```python
from build123d import *
from OCP.BRepFilletAPI import BRepFilletAPI_MakeChamfer

# Parameters (mm, degrees)
SKETCH1_R                = 2.75
BOSS_EXTRUDE1_DEPTH      = 25
CUT_EXTRUDE1_DEPTH       = 37.486298798
CUT_EXTRUDE1_DEPTH_BACK  = 37.486298798
CUT_EXTRUDE2_START       = -5
SKETCH3_R                = 6
CUT_EXTRUDE2_DEPTH       = 28.113081447
CUT_EXTRUDE3_START       = -23.75
CUT_EXTRUDE3_DEPTH       = 23.75
CUT_EXTRUDE3_START_2     = -14.426375
CUT_EXTRUDE3_2_OUTLINE_R = 2
CUT_EXTRUDE3_2_DEPTH     = 14.426375
CHAMFER1_SIZE            = 2
CHAMFER1_SIZE2           = 7.211102551
CHAMFER2_SIZE            = 0.4
SKETCH5_W                = 6
SKETCH5_H                = 4
SKETCH5_W_2              = 4
SKETCH5_H_2              = 6
BOSS_EXTRUDE2_DEPTH      = 2
CHAMFER3_SIZE            = 2


with BuildPart() as part:
    # Sketch1 → Boss-Extrude1 (new body)
    with BuildSketch(Plane.XY):
        Polygon((-10, 10), (10, 10), (10, -10), (10, -17.5), (-10, -17.5), (-10, -10), align=None)
        Circle(SKETCH1_R, mode=Mode.SUBTRACT)
    extrude(amount=BOSS_EXTRUDE1_DEPTH)

    # Sketch2 → Cut-Extrude1 (cut, two sides: drawn at the far end of the back side and taken through both)
    with BuildSketch(Plane(origin=(10, 0, 0), x_dir=(0, 0, -1), z_dir=(1, 0, 0)).offset(-CUT_EXTRUDE1_DEPTH_BACK)):
        Polygon((-5, -17.5), (0, -10), (0, -17.5), align=None)
        Polygon((-12.5, 10), (-25, -8.75), (-25, 10), align=None)
    extrude(amount=CUT_EXTRUDE1_DEPTH + CUT_EXTRUDE1_DEPTH_BACK, mode=Mode.SUBTRACT)

    # Sketch3 → Cut-Extrude2 (cut, through all)
    with BuildSketch(Plane(origin=(0, 0, 0), x_dir=(-1, 0, 0), z_dir=(0, 0, -1)).offset(CUT_EXTRUDE2_START)):
        Circle(SKETCH3_R)
    extrude(amount=-CUT_EXTRUDE2_DEPTH, mode=Mode.SUBTRACT)

    # Cut-Extrude3: read off the stored shape, not the designer's step
    # Cut-Extrude3 outline → Cut-Extrude3 (cut)
    with BuildSketch(Plane.XZ.offset(17.5).offset(CUT_EXTRUDE3_START)):
        with BuildLine():
            ThreePointArc((-10, 15), (-7.071067812, 22.071067812), (0, 25))
            Line((0, 25), (-10, 25))
            Line((-10, 25), (-10, 15))
        make_face()
        with BuildLine():
            ThreePointArc((0, 25), (7.071067812, 22.071067812), (10, 15))
            Line((10, 15), (10, 25))
            Line((10, 25), (0, 25))
        make_face()
    extrude(amount=CUT_EXTRUDE3_DEPTH, mode=Mode.SUBTRACT)

    # Cut-Extrude3 2 outline → Cut-Extrude3 2 (cut)
    with BuildSketch(Plane.XZ.offset(17.5).offset(CUT_EXTRUDE3_START_2)):
        with Locations((0, 15)):
            Circle(CUT_EXTRUDE3_2_OUTLINE_R)
    extrude(amount=CUT_EXTRUDE3_2_DEPTH, mode=Mode.SUBTRACT)

    # Chamfer1: one chamfer whose edges measure the first distance from different faces: ONE call of the kernel's chamfer builder (chamfer() names one face for all edges)
    chamfer1_edges_1 = [part.edges().sort_by_distance(p)[0] for p in [
        (-10, 10, 6.25),
        (10, 10, 6.25),
    ]]
    chamfer1_edges_2 = [part.edges().sort_by_distance(p)[0] for p in [
        (0, 10, 12.5),
    ]]
    chamfer1_side_2 = [part.faces().sort_by_distance(p)[0] for p in [
        (-9.69870073, 8.125, 13.75),
    ]]
    chamfer1 = BRepFilletAPI_MakeChamfer(part.part.solid().wrapped)
    for e in chamfer1_edges_1:
        chamfer1.Add(CHAMFER1_SIZE, e.wrapped)
    for e in chamfer1_edges_2:
        chamfer1.Add(CHAMFER1_SIZE, CHAMFER1_SIZE2, e.wrapped, chamfer1_side_2[0].wrapped)  # the first distance lies on this face
    add(Compound.cast(chamfer1.Shape()), mode=Mode.REPLACE)

    # Chamfer2
    chamfer2_edges = [part.edges().sort_by_distance(p)[0] for p in [
        (10, -17.5, 10),
        (-7.071067812, -17.5, 22.071067812),
        (-10, -17.5, 10),
    ]]
    chamfer(chamfer2_edges, length=CHAMFER2_SIZE)

    # Sketch5 → Boss-Extrude2 (add)
    with BuildSketch(Plane(origin=(0, 0, 0), x_dir=(-1, 0, 0), z_dir=(0, 0, -1))):
        with Locations((0, 8)):
            Rectangle(SKETCH5_W, SKETCH5_H)
        with Locations((8, 0)):
            Rectangle(SKETCH5_W_2, SKETCH5_H_2)
        with Locations((-8, 0)):
            Rectangle(SKETCH5_W_2, SKETCH5_H_2)
    extrude(amount=BOSS_EXTRUDE2_DEPTH)

    # Chamfer3
    chamfer3_edges = [part.edges().sort_by_distance(p)[0] for p in [
        (-8, -3, -2),
        (0, 6, -2),
        (8, -3, -2),
    ]]
    chamfer(chamfer3_edges, length=CHAMFER3_SIZE - 0.0001)  # a hair under: the kernel refuses the full size


solid = part.part
```
For this review, take the finished solid that the model builds, in its own axes (mm). A direction names the side the tool comes from. Round coordinates to 2 decimals unless told otherwise and drop trailing zeros. Write each loop counter-clockwise with the first axis right and the second up, starting at its lowest first coordinate (ties: lowest second). Pieces come first, ordered by that corner, then holes. Notation, with made-up numbers: (77.5, 34.5) -> (108.5, 34.5) arc R17 cw to (108.5, 44.5) -> close; hole circle Ø10 at (17, 89.5). An arc over 180 degrees is marked (long way). One line per question, with ' | ' between items. Start each with the question number.
1) Wall thickness on line 1 along X through (y, z) = (0, 3.15); line 2 along X through (y, z) = (0, 10.5); line 3 along Z through (x, y) = (0, -10): over which ranges is each line inside the solid? List them lowest first.
2) Mouldability with a two-part tool opening along X and no side actions: class faces 1 (the flat face through (-2.1, -2.1, 0)), 2 (the flat face through (0, 10, 2)), 3 (the flat face through (-9, 9, 5)) as +X half, -X half, draft (parallel to the pull), parting line (faces both ways), or undercut.
3) For pin 1 Ø6 at (x, y) = (-1, 0) entering from -Z; pin 2 Ø9 at (x, y) = (0, 0) entering from +Z; pin 3 Ø6.5 at (x, z) = (0, 15) entering from -Y; pin 4 Ø1 at (y, z) = (7.5, -1) entering from +X, all flat-tipped, find the tip position at first contact; note any pin that passes through.
4) Add section B-B (y = 0). Write out the cut boundary in (x, z).
5) Add section D-D (y = 4.75). Write out the cut boundary in (x, z), and give its area (3 significant figures).
6) Add section C-C (x = -1). Count the separate pieces of the cut face and the enclosed holes in it, and give its area (3 significant figures).
7) Add section A-A (y = -12.25). Write out the cut boundary in (x, z), and give its area (3 significant figures).
8) Machinability: for faces 4 (the cylindrical face through (-0.596, -2.685, 2.465)), 5 (the flat face through (-3, 8, -1)), 6 (the flat face through (-6, 1, -1)), 7 (the flat face through (3, 8, -1)), 8 (the flat face through (-8, 3, -1)), which of the approach directions +Z, -Z, +X, -X, +Y, -Y give a long, thin tool a straight path to every point of the face, cutting with its end or side? Answer none if there is none.
Reported:
1) line 1: x = -10 to -2.75, 2.75 to 10 | line 2: x = -10 to -6, 6 to 10 | line 3: z = 0 to 13, 17 to 25
2) face 1: undercut | face 2: draft | face 3: -X half
3) pin 1: stops at z = 0 | pin 2: stops at z = 5 | pin 3: stops at y = -17.5 | pin 4: stops at x = 3
4) outline: (-10, -2) -> (-6, -2) -> (-6, 0) -> (-2.75, 0) -> (-2.75, 5) -> (-6, 5) -> (-6, 19.17) -> (-9.09, 19.17) arc R10 ccw to (-10, 15) -> close; (2.75, 0) -> (6, 0) -> (6, -2) -> (10, -2) -> (10, 15) arc R10 ccw to (9.09, 19.17) -> (6, 19.17) -> (6, 5) -> (2.75, 5) -> close
5) outline: (-10, 0) -> (10, 0) -> (10, 15) arc R10 ccw to (9.95, 16) -> (3.67, 16) -> (3.67, 5) -> (-3.67, 5) -> (-3.67, 16) -> (-9.95, 16) arc R10 ccw to (-10, 15) -> close | area: 239 mm²
6) separate pieces: 3 | enclosed holes: 0 | area: 318 mm²
7) outline: (-10, 1.5) -> (10, 1.5) -> (10, 15) arc R10 ccw to (-10, 15) -> close; hole circle Ø4 at (0, 15) | area: 415 mm²
8) face 4: +Z, -Z | face 5: -Z, -X, +Y, -Y | face 6: -Z, +Y, -Y | face 7: -Z, +X, +Y, -Y | face 8: -Z, +X, -X, +Y
